```python
from build123d import *

# Parameters (mm, degrees)
BOSS_EXTRUDE1_DEPTH                      = 130
CBORE_FOR_M5_PAN_HEAD_SCREW1_D           = 5.5
CBORE_FOR_M5_PAN_HEAD_SCREW1_CBORE_D     = 11
CBORE_FOR_M5_PAN_HEAD_SCREW1_CBORE_DEPTH = 3.7
CBORE_FOR_M6_PAN_HEAD_SCREW1_D           = 6.6
CBORE_FOR_M6_PAN_HEAD_SCREW1_CBORE_D     = 13
CBORE_FOR_M6_PAN_HEAD_SCREW1_CBORE_DEPTH = 4.6


with BuildPart() as part:
    # Sketch1 → Boss-Extrude1 (new body)
    with BuildSketch(Plane.XY):
        Polygon((0, 8), (0, 0), (8, 0), (30, 0), (30, 8), (8, 8), (8, 30), (0, 30), align=None)
    extrude(amount=BOSS_EXTRUDE1_DEPTH)

    # CBORE for M5 Pan Head Screw1 (through all)
    with Locations(Plane(origin=(0, 8, 0), x_dir=(1, 0, 0), z_dir=(0, 1, 0))):
        with Locations((19, -67.160533678), (19, -37.160533678), (19, -97.160533678)):
            CounterBoreHole(CBORE_FOR_M5_PAN_HEAD_SCREW1_D / 2, CBORE_FOR_M5_PAN_HEAD_SCREW1_CBORE_D / 2, CBORE_FOR_M5_PAN_HEAD_SCREW1_CBORE_DEPTH)

    # CBORE for M6 Pan Head Screw1 (through all)
    with Locations(Plane(origin=(8, 0, 0), x_dir=(0, 0, -1), z_dir=(1, 0, 0))):
        with Locations((-110, 19), (-65, 19), (-20, 19)):
            CounterBoreHole(CBORE_FOR_M6_PAN_HEAD_SCREW1_D / 2, CBORE_FOR_M6_PAN_HEAD_SCREW1_CBORE_D / 2, CBORE_FOR_M6_PAN_HEAD_SCREW1_CBORE_DEPTH)


solid = part.part
```
Check sheet for the modelled part. Datum: model origin and axes. Units: mm. A direction names the side the tool comes from. Coordinates: 2 decimals unless noted, no trailing zeros. Loops run counter-clockwise (first coordinate to the right, second up) from the corner with the lowest first, then second, coordinate; pieces in that order, holes last.
1) Sectioned sample at D-D (y = 5.5). Record the boundary of the cut face in (x, z), and give its area (3 significant figures).
2) Gauge pin test, flat ends, axial feed: pin 1 (8 mm diameter, centred on y = 19, z = 20, fed in from -X); pin 2 (3 mm diameter, centred on y = 24, z = 49.5, fed in from +X); pin 3 (9 mm diameter, centred on x = 19, z = 37.16, fed in from +Y); pin 4 (8.5 mm diameter, centred on y = 19, z = 20, fed in from +X). Record the tip position at first contact, or that the pin passes through.
3) Sectioned sample at B-B (y = 19). Record the boundary of the cut face in (x, z).
4) Material ranges on probe 1 along Z at (x, y) = (19, 1.95); probe 2 along Z at (x, y) = (19, 6.5); probe 3 along Y at (x, z) = (1.05, 110), recorded low to high.
5) Release check for a two-part mould opening along Z. For faces 5 (the face through (8, 5, 0)), 6 (the face through (30, 4, 64)), 7 (the face through (3.4, 21, 68)) record: released by +Z, released by -Z, zero draft, split by the parting line, or undercut.
6) Sectioned sample at A-A (z = 20). Record the boundary of the cut face in (x, y).
7) Sectioned sample at C-C (x = 2). Record the boundary of the cut face in (y, z).
8) Access from +Z, -Z, +X, -X, +Y, -Y to the whole of each face (thin tool, end or side, straight path). Record for faces 1 (the face through (14, 8, 64)), 2 (the face through (1.68, 16.07, 21.52)), 3 (the face through (3.4, 22, 112)), 4 (the face through (18.284, 6.176, 61.707)).
Check sheet entries:
1. outline: (0, 0) - (30, 0) - (30, 130) - (0, 130) - close; hole circle Ø11 at (19, 37.16); hole circle Ø11 at (19, 67.16); hole circle Ø11 at (19, 97.16)
1. area: 3,610 mm2
2. pin 1: stops at x = 0
2. pin 2: stops at x = 8
2. pin 3: stops at y = 4.3
2. pin 4: stops at x = 3.4
3. outline: (0, 0) - (8, 0) - (8, 13.5) - (3.4, 13.5) - (3.4, 16.7) - (0, 16.7) - close; (0, 23.3) - (3.4, 23.3) - (3.4, 26.5) - (8, 26.5) - (8, 58.5) - (3.4, 58.5) - (3.4, 61.7) - (0, 61.7) - close; (0, 68.3) - (3.4, 68.3) - (3.4, 71.5) - (8, 71.5) - (8, 103.5) - (3.4, 103.5) - (3.4, 106.7) - (0, 106.7) - close; (0, 113.3) - (3.4, 113.3) - (3.4, 116.5) - (8, 116.5) - (8, 130) - (0, 130) - close
4. probe 1: z = 0 to 34.41, 39.91 to 64.41, 69.91 to 94.41, 99.91 to 130
4. probe 2: z = 0 to 31.66, 42.66 to 61.66, 72.66 to 91.66, 102.66 to 130
4. probe 3: y = 0 to 15.7, 22.3 to 30
5. face 5: released by -Z
5. face 6: zero draft
5. face 7: undercut
6. outline: (0, 0) - (30, 0) - (30, 8) - (8, 8) - (8, 12.5) - (3.4, 12.5) - (3.4, 15.7) - (0, 15.7) - close; (0, 22.3) - (3.4, 22.3) - (3.4, 25.5) - (8, 25.5) - (8, 30) - (0, 30) - close
7. outline: (0, 0) - (30, 0) - (30, 130) - (0, 130) - close; hole circle Ø6.6 at (19, 20); hole circle Ø6.6 at (19, 65); hole circle Ø6.6 at (19, 110)
8. face 1: +Z, -Z, +X, +Y
8. face 2: +X, -X
8. face 3: +X
8. face 4: +Y
